Here's how the part is built. I have some questions about the finished solid (model axes, mm). A direction names the side the tool comes from. Round coordinates to 2 decimals unless told otherwise and drop trailing zeros. Order: outer loops, then holes, each group sorted by start corner. A loop starts at its lowest first (then second) coordinate and runs counter-clockwise, first axis right, second up. Notation, with made-up numbers: (19.25, -3.75) - (45.25, -3.75) arc R24 ccw to (45.25, 17.25) - close; hole circle Ø6 at (3, 23.25). An arc over 180 degrees is marked (long way). Answer as a JSON object with one key per item and string values.
```python
from build123d import *

# Parameters (mm, degrees)
SKETCH1_R                = 1.1303
BOSS_EXTRUDE1_DEPTH      = 12.7
SKETCH2_W                = 9.525
SKETCH2_H                = 9.525
CUT_EXTRUDE1_DEPTH       = 13.7
BOSS_EXTRUDE2_DEPTH      = 6.35
BOSS_EXTRUDE2_DEPTH_BACK = 19.05
SKETCH5_R                = 0.6985
CUT_EXTRUDE2_DEPTH       = 4.402075722


with BuildPart() as part:
    # Sketch1 → Boss-Extrude1 (new body)
    with BuildSketch(Plane(origin=(0, 0, 0), x_dir=(1, 0, 0), z_dir=(0, 1, 0))):
        with BuildLine():
            Line((75.972924278, -6.35), (88.672924278, -6.35))
            ThreePointArc((88.672924278, -6.35), (88.9, 0), (88.672924278, 6.35))
            Line((88.672924278, 6.35), (75.972924278, 6.35))
            Line((75.972924278, 6.35), (75.972924278, -6.35))
        make_face()
        with Locations((82.322924278, 0)):
            Circle(SKETCH1_R, mode=Mode.SUBTRACT)
    extrude(amount=BOSS_EXTRUDE1_DEPTH)

    # Sketch2 → Cut-Extrude1 (cut, through all)
    with BuildSketch(Plane.XY.offset(6.35)):
        with Locations((80.735424278, 6.35)):
            Rectangle(SKETCH2_W, SKETCH2_H)
    extrude(amount=-CUT_EXTRUDE1_DEPTH, mode=Mode.SUBTRACT)

    # Sketch3 → Boss-Extrude2 (add, two sides)
    with BuildSketch(Plane(origin=(0, 12.7, 0), x_dir=(1, 0, 0), z_dir=(0, 1, 0))) as boss_extrude2_sk:
        with BuildLine():
            Line((85.497924278, -6.35), (88.672924278, -6.35))
            ThreePointArc((88.672924278, -6.35), (88.9, 0), (88.672924278, 6.35))
            Line((88.672924278, 6.35), (85.497924278, 6.35))
            Line((85.497924278, 6.35), (85.497924278, -6.35))
        make_face()
    extrude(amount=BOSS_EXTRUDE2_DEPTH)
    extrude(boss_extrude2_sk.sketch, amount=-BOSS_EXTRUDE2_DEPTH_BACK)

    # Sketch5 → Cut-Extrude2 (cut, through all)
    with BuildSketch(Plane.ZY.offset(-85.497924278)):
        with Locations((0, 15.875)):
            Circle(SKETCH5_R)
        with Locations((0, -3.175)):
            Circle(SKETCH5_R)
    extrude(amount=-CUT_EXTRUDE2_DEPTH, mode=Mode.SUBTRACT)


solid = part.part
```
1. Imagine slicing it at A-A (x = 85). List the corners of the cut face in (y, z) for me, plus the area to 3 significant figures.
Responses:
{"outline": "(0, -6.35) - (1.59, -6.35) - (1.59, 6.35) - (0, 6.35) - close; (11.11, -6.35) - (12.7, -6.35) - (12.7, 6.35) - (11.11, 6.35) - close", "area": "40.3 mm2"}
2. Imagine slicing it at B-B (z = 0). List the corners of the cut face in (x, y) for me, plus the area to 4 significant figures.
Responses:
{"outline": "(75.97, 0) - (81.19, 0) - (81.19, 1.59) - (75.97, 1.59) - close; (75.97, 11.11) - (81.19, 11.11) - (81.19, 12.7) - (75.97, 12.7) - close; (83.45, 0) - (85.5, 0) - (85.5, -2.48) - (88.9, -2.48) - (88.9, 15.18) - (85.5, 15.18) - (85.5, 12.7) - (83.45, 12.7) - (83.45, 11.11) - (85.5, 11.11) - (85.5, 1.59) - (83.45, 1.59) - close; (85.5, -6.35) - (88.9, -6.35) - (88.9, -3.87) - (85.5, -3.87) - close; (85.5, 16.57) - (88.9, 16.57) - (88.9, 19.05) - (85.5, 19.05) - close", "area": "100.0 mm2"}
3. If I drill on L1, parallel to Y at x = 87.05, z = 0; L2, parallel to Y at x = 78.5, z = -4.25; L3, parallel to X at y = 11.55, z = 0, over which ranges is the centre line in solid material (lowest first)? Write a range as [from, to].
Responses:
{"L1": "[-6.35, -3.87], [-2.48, 15.18], [16.57, 19.05]", "L2": "[0, 1.59], [11.11, 12.7]", "L3": "[75.97, 81.19], [83.45, 88.9]"}
4. Thinking about a two-plate mould opening in Z: for faces 6 (the face through (87, 19.05, 0)), 7 (the face through (86, 6, 6.35)), 8 (the face through (87, 6, -6.35)), 9 (the face through (87.175, 15.193, -0.151)), which applies, pulls with the +Z half, pulls with the -Z half, needs draft (parallel to the pull), parting line crosses it, or undercut?
Responses:
{"face 6": "needs draft", "face 7": "pulls with the +Z half", "face 8": "pulls with the -Z half", "face 9": "undercut"}
5. For P1, Ø5, axis at x = 81, z = 2, coming from the +Y side; P2, Ø5, axis at y = 7, z = -2, coming from the -X side; P3, Ø7.5, axis at x = 81.5, z = -3, coming from the -Y side; P4, Ø6, axis at x = 83, z = 0.5, coming from the -Y side, each with a flat end and sliding along its axis, tell me the tip position at first contact or that it passes through.
Responses:
{"P1": "y = 12.7", "P2": "x = 85.5", "P3": "y = 0", "P4": "y = -6.35"}
6. Imagine slicing it at D-D (y = 0.75). List the corners of the cut face in (x, z) for me, plus the area to 3 significant figures.
Responses:
{"outline": "(75.97, -6.35) - (88.67, -6.35) arc R88.9 ccw to (88.67, 6.35) - (75.97, 6.35) - close; hole circle Ø2.26 at (82.32, 0)", "area": "159 mm2"}
7. Imagine slicing it at C-C (y = 15.5). List the corners of the cut face in (x, z) for me, plus the area to 3 significant figures.
Responses:
{"outline": "(85.5, -6.35) - (88.67, -6.35) arc R88.9 ccw to (88.9, -0.59) - (85.5, -0.59) - close; (85.5, 0.59) - (88.9, 0.59) arc R88.9 ccw to (88.67, 6.35) - (85.5, 6.35) - close", "area": "38.2 mm2"}
8. For faces 1 (the face through (85.498, 15, 0)), 2 (the face through (81, 1.587, 0)), 3 (the face through (81.194, 11.895, -0.05)), 4 (the face through (85.498, -2, 0)), 5 (the face through (88.9, 6.2, 0.1)), which set-ups out of +Z, -Z, +X, -X, +Y, -Y let a thin tool reach every point of the face, with its end or its side?
Responses:
{"face 1": "+Z, -Z, -X, +Y", "face 2": "+Z, -Z, -X", "face 3": "+Y, -Y", "face 4": "+Z, -Z, -X, -Y", "face 5": "+X, +Y, -Y"}
